CAD build for the part. Positions are in the model's coordinates, mm. Face numbers are marked on the shaded views. A direction names the side the tool comes from. Coordinates: 2 decimals unless noted, no trailing zeros. Loops run counter-clockwise (first coordinate to the right, second up) from the corner with the lowest first, then second, coordinate; pieces in that order, holes last. Notation, with made-up numbers: (37, -28.5) -> (42, -28.5) arc R19 cw to (42, -8.5) -> close; hole circle Ø7 at (-13, -9). An arc over 180 degrees is marked (long way). Write each question's results on one line, items separated by ' | '.
```python
from build123d import *

# Parameters (mm, degrees)
SKETCH1_W              = 27.9
SKETCH1_H              = 21.6
BOSS_EXTRUDE1_DEPTH    = 22.6
SKETCH2_W              = 10.2
SKETCH2_H              = 19.5
CUT_EXTRUDE1_DEPTH     = 11.3
LPATTERN1_COUNT        = 2
LPATTERN1_PITCH        = 12.7
SKETCH4_W              = 3.3
SKETCH4_H              = 1.8
BOSS_EXTRUDE2_DEPTH    = 4
CHAMFER1_SIZE          = 0.5
SKETCH6_W              = 10.2
SKETCH6_H              = 11.3
CUT_EXTRUDE3_DEPTH     = 1.25
LPATTERN2_COUNT        = 2
LPATTERN2_PITCH        = 12.7
SKETCH7_R              = 3.75
BOSS_EXTRUDE3_DEPTH    = 2.5
FILLET1_R              = 1
LPATTERN3_COUNT        = 2
LPATTERN3_PITCH        = 12.7
FILLET1_OF_LPATTERN3_R = 1
FILLET2_R              = 3.5


with BuildPart() as part:
    # Sketch1 → Boss-Extrude1 (new body)
    with BuildSketch(Plane(origin=(0, 0, 0), x_dir=(1, 0, 0), z_dir=(0, 1, 0))):
        Rectangle(SKETCH1_W, SKETCH1_H)
    extrude(amount=BOSS_EXTRUDE1_DEPTH)

    # Sketch2 → Cut-Extrude1 (cut)
    with BuildSketch(Plane(origin=(0, 22.6, 0), x_dir=(1, 0, 0), z_dir=(0, 1, 0))):
        with Locations((-6.35, -1.05)):
            Rectangle(SKETCH2_W, SKETCH2_H)
    cut_extrude1 = extrude(amount=-CUT_EXTRUDE1_DEPTH, mode=Mode.SUBTRACT)

    # LPattern1: Cut-Extrude1 ×2
    with Locations(*[(i * LPATTERN1_PITCH, 0, 0) for i in range(1, LPATTERN1_COUNT)]):
        add(cut_extrude1, mode=Mode.SUBTRACT)

    # Sketch4 → Boss-Extrude2 (add)
    with BuildSketch(Plane(origin=(0, 0, 0), x_dir=(-1, 0, 0), z_dir=(0, -1, 0))):
        with Locations((-6.35, -5.2)):
            Rectangle(SKETCH4_W, SKETCH4_H)
        with Locations((6.35, 7.8)):
            Rectangle(SKETCH4_W, SKETCH4_H)
    extrude(amount=BOSS_EXTRUDE2_DEPTH)

    # Chamfer1
    chamfer1_edges = [part.edges().sort_by_distance(p)[0] for p in [
        (4.7, -4, 5.2),
        (6.35, -4, 4.3),
        (8, -4, 5.2),
        (6.35, -4, 6.1),
        (-8, -4, -7.8),
        (-6.35, -4, -8.7),
        (-4.7, -4, -7.8),
        (-6.35, -4, -6.9),
    ]]
    chamfer(chamfer1_edges, length=CHAMFER1_SIZE)

    # Sketch6 → Cut-Extrude3 (cut)
    with BuildSketch(Plane.XY.offset(10.8)):
        with Locations((-6.35, 5.65)):
            Rectangle(SKETCH6_W, SKETCH6_H)
    cut_extrude3 = extrude(amount=-CUT_EXTRUDE3_DEPTH, mode=Mode.SUBTRACT)

    # LPattern2: Cut-Extrude3 ×2
    with Locations(*[(i * LPATTERN2_PITCH, 0, 0) for i in range(1, LPATTERN2_COUNT)]):
        add(cut_extrude3, mode=Mode.SUBTRACT)

    # Sketch7 → Boss-Extrude3 (add)
    with BuildSketch(Plane(origin=(0, 11.3, 0), x_dir=(1, 0, 0), z_dir=(0, 1, 0))):
        with Locations(Location((-6.35, 1.3, 0), (0, 0, 90))):
            Circle(SKETCH7_R)
    boss_extrude3 = extrude(amount=BOSS_EXTRUDE3_DEPTH)

    # Fillet1
    fillet1_edges = [part.edges().sort_by_distance(p)[0] for p in [
        (-6.35, 13.8, 2.45),
    ]]
    fillet(fillet1_edges, radius=FILLET1_R)

    # LPattern3: Boss-Extrude3 ×2
    with Locations(*[(i * LPATTERN3_PITCH, 0, 0) for i in range(1, LPATTERN3_COUNT)]):
        add(boss_extrude3)

    # Fillet1 of LPattern3
    fillet1_of_lpattern3_edges = [part.edges().sort_by_distance(p)[0] for p in [
        (6.35, 13.8, 2.45),
    ]]
    fillet(fillet1_of_lpattern3_edges, radius=FILLET1_OF_LPATTERN3_R)

    # Fillet2
    fillet2_edges = [part.edges().sort_by_distance(p)[0] for p in [
        (-12.7, 22.6, 10.8),
        (0, 22.6, 10.8),
        (12.7, 22.6, 10.8),
    ]]
    fillet(fillet2_edges, radius=FILLET2_R)


solid = part.part
```
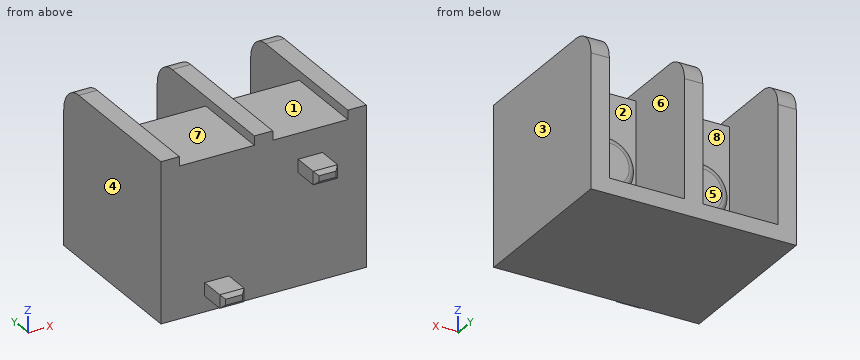
Q1. Cut at C-C on x = -6.35. Write the cut outline in (y, z).
Results are:
outline: (-4, -8.2) -> (-3.5, -8.7) -> (0, -8.7) -> (0, -10.8) -> (22.6, -10.8) -> (22.6, -8.7) -> (11.3, -8.7) -> (11.3, -5.05) -> (12.8, -5.05) arc R1 ccw to (13.8, -4.05) -> (13.8, 1.45) arc R1 ccw to (12.8, 2.45) -> (11.3, 2.45) -> (11.3, 9.55) -> (0, 9.55) -> (0, -6.9) -> (-3.5, -6.9) -> (-4, -7.4) -> close
Q2. Cut at A-A on z = -1.3. Write the cut outline in (x, y), and give its area (3 significant figures).
Results are:
outline: (-13.95, 0) -> (13.95, 0) -> (13.95, 22.6) -> (11.45, 22.6) -> (11.45, 11.3) -> (10.1, 11.3) -> (10.1, 12.8) arc R1 ccw to (9.1, 13.8) -> (3.6, 13.8) arc R1 ccw to (2.6, 12.8) -> (2.6, 11.3) -> (1.25, 11.3) -> (1.25, 22.6) -> (-1.25, 22.6) -> (-1.25, 11.3) -> (-2.6, 11.3) -> (-2.6, 12.8) arc R1 ccw to (-3.6, 13.8) -> (-9.1, 13.8) arc R1 ccw to (-10.1, 12.8) -> (-10.1, 11.3) -> (-11.45, 11.3) -> (-11.45, 22.6) -> (-13.95, 22.6) -> close | area: 437 mm^2
Q3. Cut at D-D on z = 6.5. Write the cut outline in (x, y).
Results are:
outline: (-13.95, 0) -> (13.95, 0) -> (13.95, 22.6) -> (11.45, 22.6) -> (11.45, 11.3) -> (1.25, 11.3) -> (1.25, 22.6) -> (-1.25, 22.6) -> (-1.25, 11.3) -> (-11.45, 11.3) -> (-11.45, 22.6) -> (-13.95, 22.6) -> close
Q4. Drop flat-ended pins along their axis: pin 1 (0.9 mm diameter, centred on y = -1.5, z = -7.5, fed in from -X); pin 2 (2 mm diameter, centred on y = -1.5, z = -8, fed in from +X); pin 3 (6 mm diameter, centred on x = -5.5, z = -1, fed in from +Y); pin 4 (11 mm diameter, centred on x = -7, y = 3, fed in from +Z). Give the stop position or say it passes through.
Results are:
pin 1: x = -8 | pin 2: x = -4.7 | pin 3: y = 13.8 | pin 4: z = 10.8
Q5. Pull direction Z, two halves, no side cores. Call the marked faces 6, 7 and 8: +Z half, -Z half, draft (parallel to the pull), parting line (faces both ways), or undercut.
Results are:
face 6: draft | face 7: +Z half | face 8: undercut
Q6. Which spindle directions (+Z, -Z, +X, -X, +Y, -Y) get a long thin tool onto all of the face, cutting with end or side? Do the marked faces 1, 2, 3, 4 and 5. Say none if no direction does.
Results are:
face 1: +Z, +Y, -Y | face 2: +Y | face 3: +Z, -Z, +X, +Y, -Y | face 4: +Z, -Z, -X, +Y, -Y | face 5: +Z, +Y
Q7. Cut at B-B on y = 8.5. Write the cut outline in (x, z).
Results are:
outline: (-13.95, -10.8) -> (13.95, -10.8) -> (13.95, 10.8) -> (11.45, 10.8) -> (11.45, 9.55) -> (1.25, 9.55) -> (1.25, 10.8) -> (-1.25, 10.8) -> (-1.25, 9.55) -> (-11.45, 9.55) -> (-11.45, 10.8) -> (-13.95, 10.8) -> close
Q8. Wall check: L1, parallel to X at y = 19.25, z = 5; L2, parallel to Y at x = 6.5, z = -6.5. Give the ranges that are in metal, low to high. Write a range as from..to.
Results are:
L1: -13.95..-11.45, -1.25..1.25, 11.45..13.95 | L2: 0..11.3
